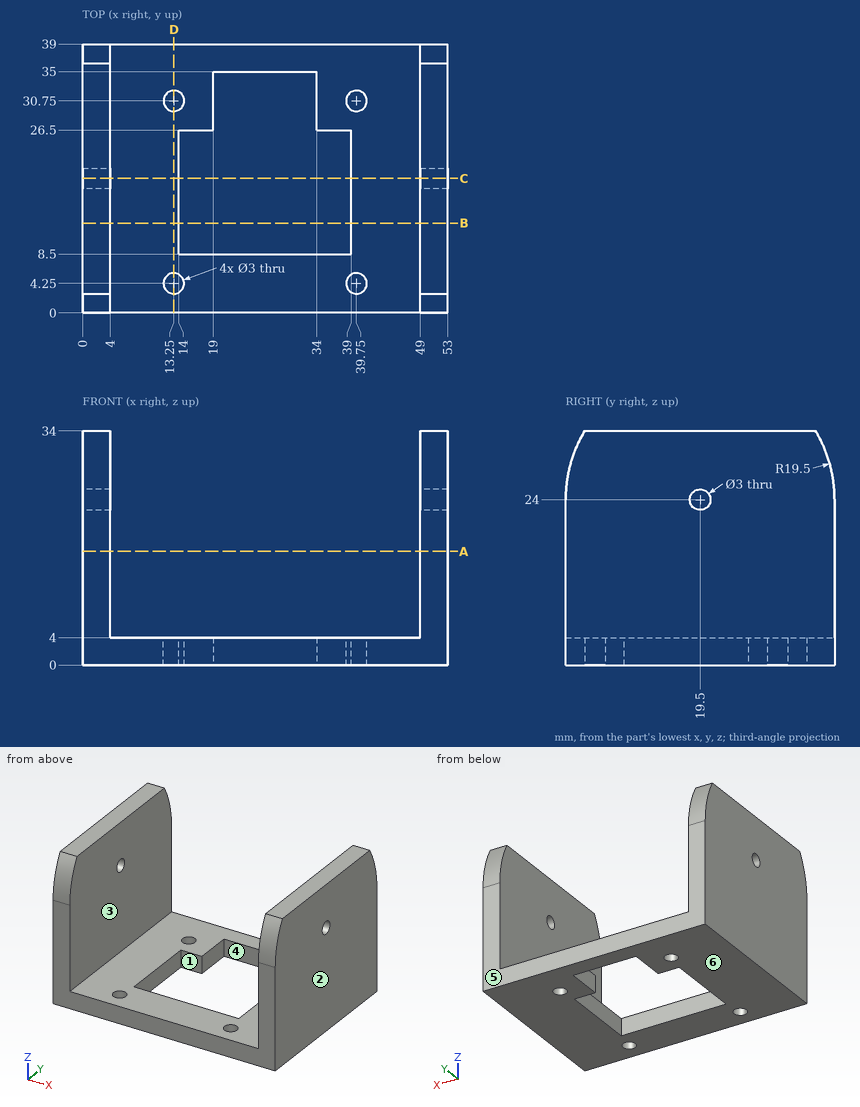
Geometry check sheet. Reference: drawing and pictorial views, mm from the part's lowest x, y, z. A direction names the side the tool comes from. Coordinates: 2 decimals unless noted, no trailing zeros. Write each loop counter-clockwise with the first axis right and the second up, starting at its lowest first coordinate (ties: lowest second). Pieces come first, ordered by that corner, then holes. Notation, with made-up numbers: (31, 14.25) -> (87, 14.25) arc R29 cw to (87, 43.25) -> close; hole circle Ø1 at (8.25, 41). An arc over 180 degrees is marked (long way). Use a Markdown table: item, result.
1. Scan lines: line 1 along Y through (x, z) = (13.25, 2.3); line 2 along X through (y, z) = (32, 5.5); line 3 along X through (y, z) = (30, 2). Record each from-to range of solid material in increasing order.
Reported:
| item | result |
|---|---|
| line 1 | y = 0 to 2.75, 5.75 to 29.25, 32.25 to 39 |
| line 2 | x = 0 to 4, 49 to 53 |
| line 3 | x = 0 to 11.95, 14.55 to 19, 34 to 38.45, 41.05 to 53 |
2. Tool access check on the marked faces 1, 2 and 3. Record the directions out of +Z, -Z, +X, -X, +Y, -Y that give a thin tool (end or side, any length) a straight path to the whole face; none if there is none.
Reported:
| item | result |
|---|---|
| face 1 | +Z, -Z |
| face 2 | +Z, -Z, +X, +Y, -Y |
| face 3 | +Z, +Y, -Y |
3. Sectioned sample at D-D (x = 13.25). Enter the section's corners in (y, z).
Reported:
| item | result |
|---|---|
| outline | (0, 0) -> (2.75, 0) -> (2.75, 4) -> (0, 4) -> close; (5.75, 0) -> (29.25, 0) -> (29.25, 4) -> (5.75, 4) -> close; (32.25, 0) -> (39, 0) -> (39, 4) -> (32.25, 4) -> close |
4. Go/stop test with flat-tipped pins: pin 1 Ø8 at (x, y) = (20.5, 4.5) entering from -Z; pin 2 Ø3 at (x, y) = (34.5, 4) entering from +Z. Record where each tip stops, or that it passes through.
Reported:
| item | result |
|---|---|
| pin 1 | stops at z = 0 |
| pin 2 | stops at z = 4 |
5. Sectioned sample at B-B (y = 13). Enter the section's corners in (x, z).
Reported:
| item | result |
|---|---|
| outline | (0, 0) -> (14, 0) -> (14, 4) -> (4, 4) -> (4, 34) -> (0, 34) -> close; (39, 0) -> (53, 0) -> (53, 34) -> (49, 34) -> (49, 4) -> (39, 4) -> close |
6. Sectioned sample at C-C (y = 19.5). Enter the section's corners in (x, z).
Reported:
| item | result |
|---|---|
| outline | (0, 0) -> (14, 0) -> (14, 4) -> (4, 4) -> (4, 22.5) -> (0, 22.5) -> close; (0, 25.5) -> (4, 25.5) -> (4, 34) -> (0, 34) -> close; (39, 0) -> (53, 0) -> (53, 22.5) -> (49, 22.5) -> (49, 4) -> (39, 4) -> close; (49, 25.5) -> (53, 25.5) -> (53, 34) -> (49, 34) -> close |
7. Sectioned sample at A-A (z = 16.5). Enter the section's corners in (x, y).
Reported:
| item | result |
|---|---|
| outline | (0, 0) -> (4, 0) -> (4, 39) -> (0, 39) -> close; (49, 0) -> (53, 0) -> (53, 39) -> (49, 39) -> close |
8. Release check for a two-part mould opening along Y. For the marked faces 4, 5 and 6 record: pulls with the +Y half, pulls with the -Y half, needs draft (parallel to the pull), parting line crosses it, or undercut.
Reported:
| item | result |
|---|---|
| face 4 | undercut |
| face 5 | pulls with the +Y half |
| face 6 | needs draft |
